Answer from the drawing. Dimensions are ordinates in mm from the lowest x, y and z of the part. A direction names the side the tool comes from. Give positions to 0.01 mm unless a question says otherwise; leave off trailing zeros. Loops run counter-clockwise (first coordinate to the right, second up) from the corner with the lowest first, then second, coordinate; pieces in that order, holes last. Notation, with made-up numbers: (61.25, -27) - (89.25, -27) arc R7 ccw to (89.25, -22) - close; hole circle Ø8 at (-1, 24.25). An arc over 180 degrees is marked (long way). Write each question's results on one line, items separated by ' | '. Start each with the question number.
Q1. The part is cut by section D-D, the plane y = 3.5. Write down the section's boundary in (x, z).
Q2. Given pin 1 (4 mm diameter, centred on y = 9, z = 9.5, fed in from +X); pin 2 (5 mm diameter, centred on x = 7.5, y = 8, fed in from +Z), each flat-ended and moving along its own axis, determine where each tip first touches the part or whether it passes through.
Q3. The part is cut by section A-A, the plane x = 6.5. Write down the section's boundary in (y, z), plus the area to 3 significant figures.
Q4. Find the intervals of material crossed by line 1 (Y direction, x = 6.5, z = 2.15); line 2 (Y direction, x = 1.45, z = 7); line 3 (X direction, y = 4.75, z = 15.5), in increasing order. Write a range as from..to.
Q5. The part is cut by section C-C, the plane y = 6. Write down the section's boundary in (x, z).
Q6. For the marked faces 1 and 2, determine the directions among +Z, -Z, +X, -X, +Y, -Y from which every point of the face is accessible in a straight line to the end or side of a thin tool.
Q7. The part is cut by section B-B, the plane z = 7. Write down the section's boundary in (x, y), plus the area to 3 significant figures.
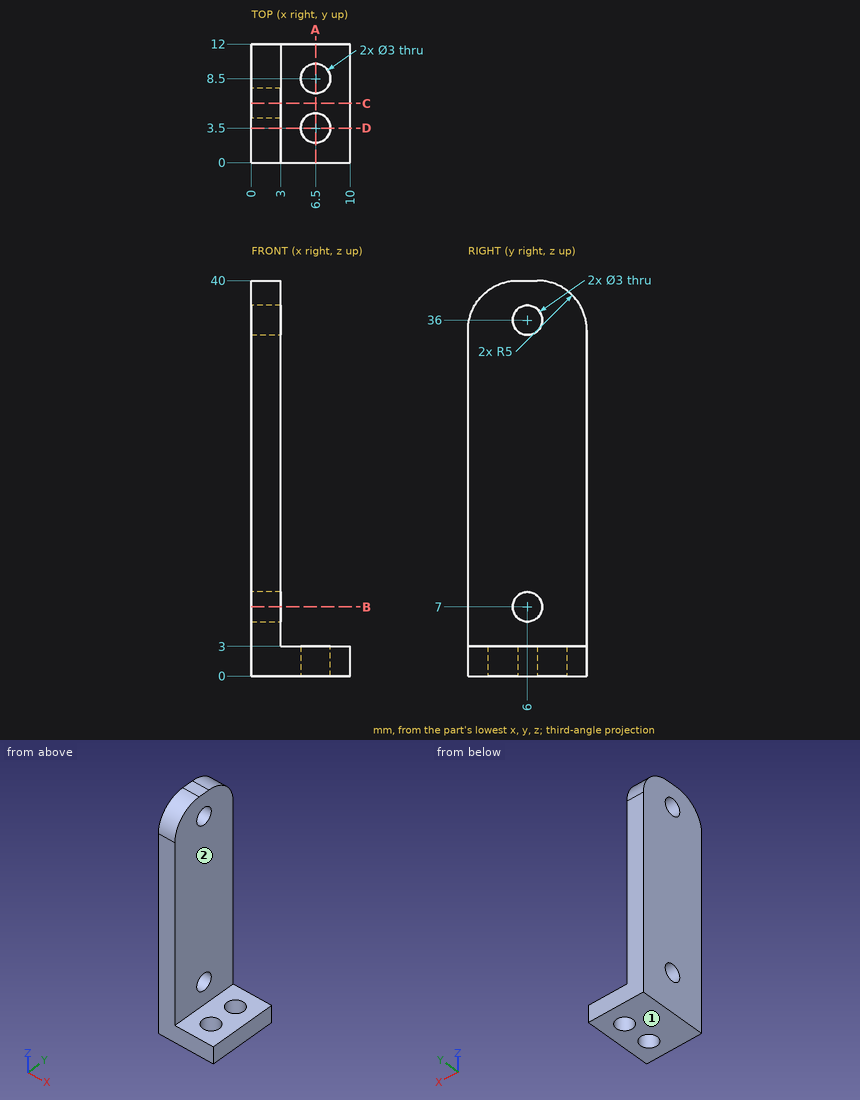
Check sheet entries:
1) outline: (0, 0) - (5, 0) - (5, 3) - (3, 3) - (3, 39.77) - (0, 39.77) - close; (8, 0) - (10, 0) - (10, 3) - (8, 3) - close
2) pin 1: stops at x = 3 | pin 2: stops at z = 3
3) outline: (0, 0) - (2, 0) - (2, 3) - (0, 3) - close; (5, 0) - (7, 0) - (7, 3) - (5, 3) - close; (10, 0) - (12, 0) - (12, 3) - (10, 3) - close | area: 18.0 mm^2
4) line 1: y = 0..2, 5..7, 10..12 | line 2: y = 0..4.5, 7.5..12 | line 3: x = 0..3
5) outline: (0, 0) - (10, 0) - (10, 3) - (3, 3) - (3, 5.5) - (0, 5.5) - close; (0, 8.5) - (3, 8.5) - (3, 34.5) - (0, 34.5) - close; (0, 37.5) - (3, 37.5) - (3, 40) - (0, 40) - close
6) face 1: -Z, +X, -X, +Y, -Y | face 2: +Z, +X, +Y, -Y
7) outline: (0, 0) - (3, 0) - (3, 4.5) - (0, 4.5) - close; (0, 7.5) - (3, 7.5) - (3, 12) - (0, 12) - close | area: 27.0 mm^2
